from build123d import *

# Parameters (mm, degrees)
F0_R     = 38.1
F1_DEPTH = 15.875
F3_DEPTH = 238.50152
F4_R     = 12.7
F5_DEPTH = 25.4
F6_R     = 12.7
F7_DEPTH = 25.4


with BuildPart() as f1:
    # F0 (on Front) → F1 (new body, symmetric)
    with BuildSketch(Plane.XZ):
        with BuildLine():
            Line((88.9, 76.2), (0, 76.2))
            ThreePointArc((0, 76.2), (-76.2, 0), (0, -76.2))
            Line((0, -76.2), (88.9, -76.2))
            Line((88.9, -76.2), (88.9, 76.2))
        make_face()
        Circle(F0_R, mode=Mode.SUBTRACT)
    extrude(amount=F1_DEPTH, both=True)

    # F2 (on face) → F3 (cut, symmetric)
    with BuildSketch(Plane.XY.offset(76.2)):
        with BuildLine():
            Line((50.8, 6.35), (0, 6.35))
            ThreePointArc((0, 6.35), (-6.35, 0), (0, -6.35))
            Line((0, -6.35), (50.8, -6.35))
            ThreePointArc((50.8, -6.35), (57.15, 0), (50.8, 6.35))
        make_face()
    extrude(amount=F3_DEPTH, both=True, mode=Mode.SUBTRACT)

    # F4 (on face) → F5 (join)
    with BuildSketch(Plane.XY.offset(76.2)):
        with BuildLine():
            Line((88.9, -15.875), (94.472131, -15.875))
            ThreePointArc((94.472131, -15.875), (90.333483, -8.412257), (88.9, 0))
            Line((88.9, 0), (88.9, -15.875))
        make_face()
        with BuildLine():
            ThreePointArc((94.472131, -15.875), (122.712257, -23.966517), (139.7, 0))
            ThreePointArc((139.7, 0), (122.712257, 23.966517), (94.472131, 15.875))
            ThreePointArc((94.472131, 15.875), (90.333483, 8.412257), (88.9, 0))
            ThreePointArc((88.9, 0), (90.333483, -8.412257), (94.472131, -15.875))
        make_face()
        with Locations((114.3, 0)):
            Circle(F4_R, mode=Mode.SUBTRACT)
        with BuildLine():
            ThreePointArc((88.9, 0), (90.333483, 8.412257), (94.472131, 15.875))
            Line((94.472131, 15.875), (88.9, 15.875))
            Line((88.9, 15.875), (88.9, 0))
        make_face()
    extrude(amount=-F5_DEPTH)

    # F6 (on face) → F7 (join)
    with BuildSketch(Plane(origin=(0, 0, -76.2), x_dir=(1, 0, 0), z_dir=(0, 0, -1))):
        with BuildLine():
            ThreePointArc((94.472131, -15.875), (122.712257, -23.966517), (139.7, 0))
            ThreePointArc((139.7, 0), (122.712257, 23.966517), (94.472131, 15.875))
            ThreePointArc((94.472131, 15.875), (90.333483, 8.412257), (88.9, 0))
            ThreePointArc((88.9, 0), (90.333483, -8.412257), (94.472131, -15.875))
        make_face()
        with Locations((114.3, 0)):
            Circle(F6_R, mode=Mode.SUBTRACT)
        with BuildLine():
            ThreePointArc((88.9, 0), (90.333483, 8.412257), (94.472131, 15.875))
            Line((94.472131, 15.875), (88.9, 15.875))
            Line((88.9, 15.875), (88.9, 0))
        make_face()
        with BuildLine():
            Line((88.9, -15.875), (94.472131, -15.875))
            ThreePointArc((94.472131, -15.875), (90.333483, -8.412257), (88.9, 0))
            Line((88.9, 0), (88.9, -15.875))
        make_face()
    extrude(amount=-F7_DEPTH)


solid = f1.part
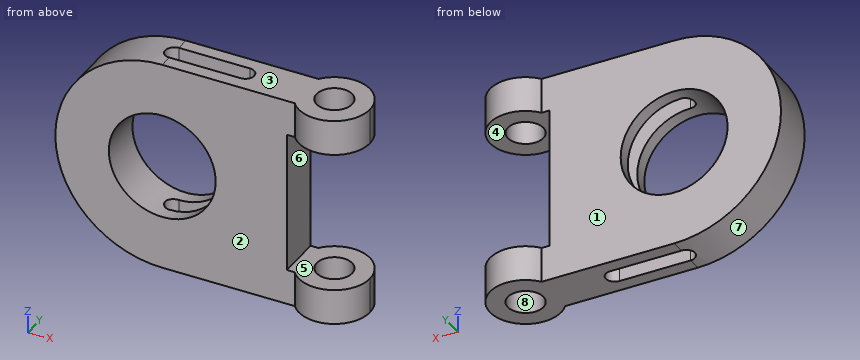
Here's how the part is built. I have some questions about the finished solid (model axes, mm). Face numbers are marked on the shaded views. A direction names the side the tool comes from. Coordinates: 2 decimals unless noted, no trailing zeros. Write each loop counter-clockwise with the first axis right and the second up, starting at its lowest first coordinate (ties: lowest second). Pieces come first, ordered by that corner, then holes.
Item 1: If I drill on line 1 (Y direction, x = 114, z = -66); line 2 (X direction, y = 0, z = -61.75); line 3 (X direction, y = 0, z = -70), over which ranges is the centre line in solid material (lowest first)?
Item 2: On a 3-axis mill with a long thin cutter (end or side, diameter ignored), from which of +Z, -Z, +X, -X, +Y, -Y can I reach the whole of each face in a straight line? I mean the marked faces 1, 2, 3 and 4. Say none if no direction works.
Item 3: I want a section at C-C on z = 0. Write out the boundary of the cut face in (x, y) (3 decimals).
Item 4: I want a section at D-D on x = 47. Write out the boundary of the cut face in (y, z) (3 decimals), and give its area (3 significant figures).
Item 5: If we mould it in two halves opening along X, with no side actions, what happens to the marked faces 5, 6, 7 and 8? For each: +X half, -X half, draft (parallel to the pull), parting line (faces both ways), or undercut.
Item 6: I want a section at B-B on y = 10.5. Write out the boundary of the cut face in (x, z).
Item 7: Will these pins go through, and if not, where does the flat tip stop? pin 1 (20.5 mm diameter, centred on x = 114.3, y = 0, fed in from -Z); pin 2 (2 mm diameter, centred on y = -2, z = 20, fed in from +X); pin 3 (12 mm diameter, centred on x = -28, y = -14.5, fed in from -Z); pin 4 (5 mm diameter, centred on y = 1.5, z = -34, fed in from -X).
Item 8: I want a section at A-A on x = 114.3. Write out the boundary of the cut face in (y, z), and give its area (3 significant figures).
Findings below:
1. line 1: y = -25.4 to -12.7, 12.7 to 25.4
1. line 2: x = -44.65 to -6.35, 57.15 to 101.6, 127 to 139.7
1. line 3: x = -30.11 to -6.35, 57.15 to 101.6, 127 to 139.7
2. face 1: +Z, -Z, -X, +Y
2. face 2: +Z, -Z, -X, -Y
2. face 3: +Z, +X, -X, +Y, -Y
2. face 4: +X, +Y, -Y
3. outline: (-76.2, -15.875) - (-38.1, -15.875) - (-38.1, 15.875) - (-76.2, 15.875) - close; (38.1, -15.875) - (88.9, -15.875) - (88.9, 15.875) - (38.1, 15.875) - (38.1, 6.35) - (50.8, 6.35) arc R6.35 cw to (50.8, -6.35) - (38.1, -6.35) - close
4. outline: (-15.875, -76.2) - (-6.35, -76.2) - (-6.35, 76.2) - (-15.875, 76.2) - close; (6.35, -76.2) - (15.875, -76.2) - (15.875, 76.2) - (6.35, 76.2) - close
4. area: 2,900 mm2
5. face 5: draft
5. face 6: +X half
5. face 7: -X half
5. face 8: undercut
6. outline: (0, -76.2) - (107.16, -76.2) - (107.16, -50.8) - (88.9, -50.8) - (88.9, 50.8) - (107.16, 50.8) - (107.16, 76.2) - (0, 76.2) arc R76.2 ccw to start; (121.44, -76.2) - (137.43, -76.2) - (137.43, -50.8) - (121.44, -50.8) - close; (121.44, 50.8) - (137.43, 50.8) - (137.43, 76.2) - (121.44, 76.2) - close; hole circle Ø76.2 at (0, 0)
7. pin 1: passes through
7. pin 2: stops at x = 88.9
7. pin 3: stops at z = -72.96
7. pin 4: stops at x = -69.38
8. outline: (-25.4, -76.2) - (-12.7, -76.2) - (-12.7, -50.8) - (-25.4, -50.8) - close; (-25.4, 50.8) - (-12.7, 50.8) - (-12.7, 76.2) - (-25.4, 76.2) - close; (12.7, -76.2) - (25.4, -76.2) - (25.4, -50.8) - (12.7, -50.8) - close; (12.7, 50.8) - (25.4, 50.8) - (25.4, 76.2) - (12.7, 76.2) - close
8. area: 1,290 mm2
